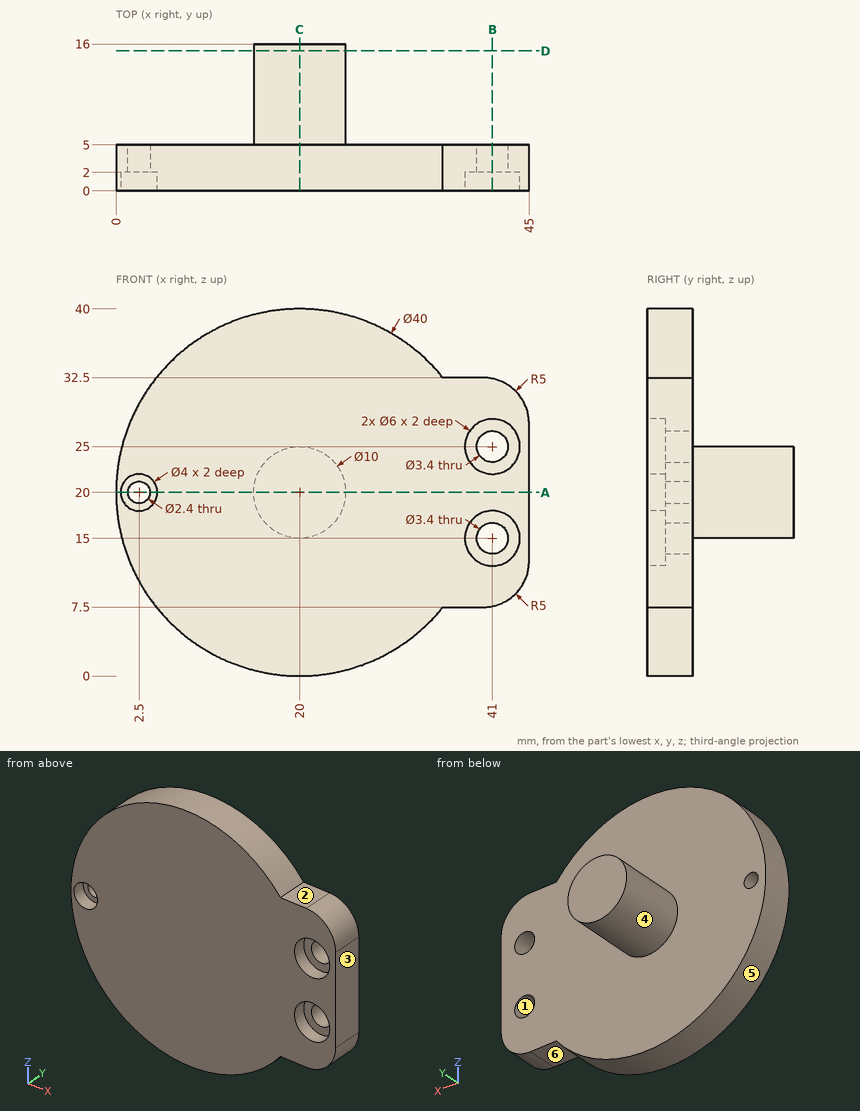
For this review, use the dimensioned drawing (mm, ordinates from the lowest corner) and the shaded views. A direction names the side the tool comes from. Round coordinates to 2 decimals unless told otherwise and drop trailing zeros. Loops run counter-clockwise (first coordinate to the right, second up) from the corner with the lowest first, then second, coordinate; pieces in that order, holes last. Notation, with made-up numbers: M 3.5,14.5 L 48.5,14.5 A10 ccw 48.5,18.5 Z; hole C 38,30 d9. An arc over 180 degrees is marked long. Answer as a JSON object with one key per item and string values.
(1) Take a section at C-C on x = 20. Give the boundary of the cut face in (y, z), and give its area (3 significant figures).
Resolved:
{"outline": "M 0,0 L 5,0 L 5,15 L 16,15 L 16,25 L 5,25 L 5,40 L 0,40 Z", "area": "310 mm²"}
(2) Take a section at B-B on x = 41. Give the boundary of the cut face in (y, z).
Resolved:
{"outline": "M 0,7.6 L 5,7.6 L 5,13.3 L 2,13.3 L 2,12 L 0,12 Z; M 0,18 L 2,18 L 2,16.7 L 5,16.7 L 5,23.3 L 2,23.3 L 2,22 L 0,22 Z; M 0,28 L 2,28 L 2,26.7 L 5,26.7 L 5,32.4 L 0,32.4 Z"}
(3) Tool access review of the marked faces 4, 5 and 6: name each direction out of +Z, -Z, +X, -X, +Y, -Y from which nothing blocks a thin tool from reaching the whole face with its end or side.
Resolved:
{"face 4": "+Y", "face 5": "+Y, -Y", "face 6": "-Z, +X, +Y, -Y"}
(4) Take a section at A-A on z = 20. Give the boundary of the cut face in (x, y).
Resolved:
{"outline": "M 0,0 L 0.5,0 L 0.5,2 L 1.3,2 L 1.3,5 L 0,5 Z; M 3.7,2 L 4.5,2 L 4.5,0 L 45,0 L 45,5 L 25,5 L 25,16 L 15,16 L 15,5 L 3.7,5 Z"}
(5) Draft analysis for pull direction X (two halves, no side actions). For the marked faces 1, 2 and 3, state which applies: released by +X, released by -X, zero draft, split by the parting line, or undercut.
Resolved:
{"face 1": "undercut", "face 2": "zero draft", "face 3": "released by +X"}
(6) To check wall thickness, follow line 1 along Y through (x, z) = (16.5, 25.5); line 2 along X through (y, z) = (1.25, 13.5); line 3 along X through (y, z) = (11.25, 23.5). State the ranges of each line that lie inside material, in increasing order.
Resolved:
{"line 1": "0 to 5", "line 2": "1.09 to 38.4, 43.6 to 45", "line 3": "16.43 to 23.57"}
(7) Take a section at D-D on y = 15.25. Give the boundary of the cut face in (x, z).
Resolved:
{"outline": "C 20,20 d10"}
(8) Clearance check with flat-ended pins moving along their axes: P1, Ø2, axis at x = 18, z = 29.5, coming from the +Y side; P2, Ø1, axis at x = 28, z = 9, coming from the -Y side; P3, Ø2.5, axis at x = 41, z = 15, coming from the +Y side; P4, Ø1, axis at y = 7.5, z = 23.5, coming from the -X side. State where each tip first meets the part, or that it passes through.
Resolved:
{"P1": "y = 5", "P2": "y = 0", "P3": "through", "P4": "x = 16"}
